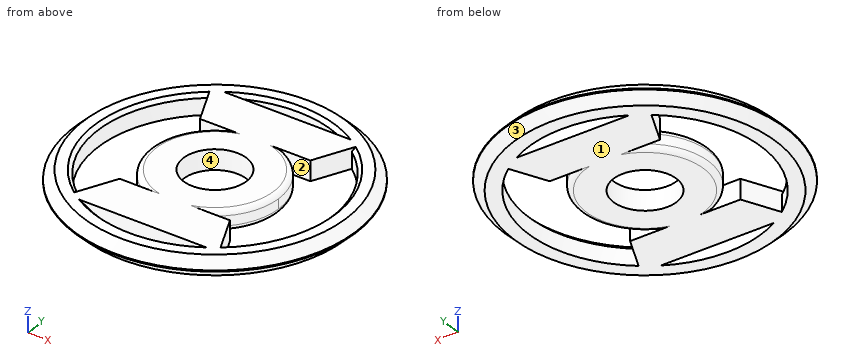
```python
from build123d import *

# Parameters (mm, degrees)
F0_R         = 49.0432335283
F0_R_2       = 10.9855
F1_DEPTH     = 6.985
F2_T4_ANGLE  = 164.4789683114
F2_T10_ANGLE = 164.4789683114
F2_T16_ANGLE = 164.4789683114
F2_T22_ANGLE = 164.4789683114
F3_T4_ANGLE  = 113.2359316918
F3_T10_ANGLE = 67.3888483325
F3_T15_ANGLE = 113.2359316918
F3_T21_ANGLE = 67.3888483325
F4_SIZE      = 3.302


# Not quite as in the source:
# - a fillet or chamfer that OpenCascade refuses, or shapes differently, is made with other operations: its cross-section is extruded or revolved along the edge and cut away or added


with BuildPart() as f1:
    # F0 (on Top) → F1 (new body)
    with BuildSketch(Plane.XY):
        Circle(F0_R)
        with BuildLine():
            Line((26.67, 35.56), (25.0451862182, 32.0755756003))
            ThreePointArc((25.0451862182, 32.0755756003), (36.5740630803, 17.8449380104), (40.6952565147, 0))
            ThreePointArc((40.6952565147, 0), (36.5738989199, -17.8452744611), (25.0445960757, -32.0760363854))
            Line((25.0445960757, -32.0760363854), (26.67, -35.56))
            Line((26.67, -35.56), (19.7886407516, -35.56))
            ThreePointArc((19.7886407516, -35.56), (0, -40.6952565147), (-19.7886407516, -35.56))
            Line((-19.7886407516, -35.56), (-26.67, -35.56))
            Line((-26.67, -35.56), (-25.0445960757, -32.0760363854))
            ThreePointArc((-25.0445960757, -32.0760363854), (-40.695256513, -0.0003743631), (-25.0451862182, 32.0755756003))
            Line((-25.0451862182, 32.0755756003), (-26.67, 35.56))
            Line((-26.67, 35.56), (-19.7886407516, 35.56))
            ThreePointArc((-19.7886407516, 35.56), (0, 40.6952565147), (19.7886407516, 35.56))
            Line((19.7886407516, 35.56), (26.67, 35.56))
        make_face(mode=Mode.SUBTRACT)
        with BuildLine():
            ThreePointArc((-10.1860168797, 19.7533714876), (0, 22.225), (10.1860168797, 19.7533714876))
            Line((10.1860168797, 19.7533714876), (19.299248075, 19.7533714876))
            Line((19.299248075, 19.7533714876), (25.0451862182, 32.0755756003))
            ThreePointArc((25.0451862182, 32.0755756003), (22.4845127485, 33.9197669399), (19.7886407516, 35.56))
            Line((19.7886407516, 35.56), (-19.7886407516, 35.56))
            ThreePointArc((-19.7886407516, 35.56), (-22.4845127485, 33.9197669399), (-25.0451862182, 32.0755756003))
            Line((-25.0451862182, 32.0755756003), (-19.299248075, 19.7533714876))
            Line((-19.299248075, 19.7533714876), (-10.1860168797, 19.7533714876))
        make_face()
        with BuildLine():
            Line((-26.67, 35.56), (-25.0451862182, 32.0755756003))
            ThreePointArc((-25.0451862182, 32.0755756003), (-22.4845127485, 33.9197669399), (-19.7886407516, 35.56))
            Line((-19.7886407516, 35.56), (-26.67, 35.56))
        make_face()
        with BuildLine():
            ThreePointArc((19.7886407516, 35.56), (22.4845127485, 33.9197669399), (25.0451862182, 32.0755756003))
            Line((25.0451862182, 32.0755756003), (26.67, 35.56))
            Line((26.67, 35.56), (19.7886407516, 35.56))
        make_face()
        with BuildLine():
            ThreePointArc((10.1708209875, -19.7612), (18.9736280327, -11.5737662097), (22.225, 0))
            ThreePointArc((22.225, 0), (18.9780774863, 11.5664687751), (10.1860168797, 19.7533714876))
            Line((10.1860168797, 19.7533714876), (0, 19.7533714876))
            Line((0, 19.7533714876), (-10.1860168797, 19.7533714876))
            ThreePointArc((-10.1860168797, 19.7533714876), (-22.2249983566, -0.0085469402), (-10.1708209875, -19.7612))
            Line((-10.1708209875, -19.7612), (0, -19.7612))
            Line((0, -19.7612), (10.1708209875, -19.7612))
        make_face()
        Circle(F0_R_2, mode=Mode.SUBTRACT)
        with BuildLine():
            Line((0, 19.7533714876), (10.1860168797, 19.7533714876))
            ThreePointArc((10.1860168797, 19.7533714876), (0, 22.225), (-10.1860168797, 19.7533714876))
            Line((-10.1860168797, 19.7533714876), (0, 19.7533714876))
        make_face()
        with BuildLine():
            Line((19.299248075, -19.7612), (10.1708209875, -19.7612))
            ThreePointArc((10.1708209875, -19.7612), (0, -22.225), (-10.1708209875, -19.7612))
            Line((-10.1708209875, -19.7612), (-19.299248075, -19.7612))
            Line((-19.299248075, -19.7612), (-25.0445960757, -32.0760363854))
            ThreePointArc((-25.0445960757, -32.0760363854), (-22.4842007134, -33.9199737776), (-19.7886407516, -35.56))
            Line((-19.7886407516, -35.56), (19.7886407516, -35.56))
            ThreePointArc((19.7886407516, -35.56), (22.4842007134, -33.9199737776), (25.0445960757, -32.0760363854))
            Line((25.0445960757, -32.0760363854), (19.299248075, -19.7612))
        make_face()
        with BuildLine():
            ThreePointArc((-10.1708209875, -19.7612), (0, -22.225), (10.1708209875, -19.7612))
            Line((10.1708209875, -19.7612), (0, -19.7612))
            Line((0, -19.7612), (-10.1708209875, -19.7612))
        make_face()
        with BuildLine():
            ThreePointArc((-19.7886407516, -35.56), (-22.4842007134, -33.9199737776), (-25.0445960757, -32.0760363854))
            Line((-25.0445960757, -32.0760363854), (-26.67, -35.56))
            Line((-26.67, -35.56), (-19.7886407516, -35.56))
        make_face()
        with BuildLine():
            Line((26.67, -35.56), (25.0445960757, -32.0760363854))
            ThreePointArc((25.0445960757, -32.0760363854), (22.4842007134, -33.9199737776), (19.7886407516, -35.56))
            Line((19.7886407516, -35.56), (26.67, -35.56))
        make_face()
    extrude(amount=F1_DEPTH)

    # F2: fillet of radius 1.778 on 4 edges, made by hand


with BuildPart() as f2_tool2:
    # F2_s3 → F2_t4 (revolve)
    with BuildSketch(Plane(origin=(0, 0, 0), x_dir=(0, 0, 1), z_dir=(0.9907891286, 0.1354138197, 0))):
        with BuildLine():
            ThreePointArc((5.207, -22.225), (6.4642358569, -21.7042358569), (6.985, -20.447))
            Line((6.985, -20.447), (6.985, -22.225))
            Line((6.985, -22.225), (5.207, -22.225))
        make_face()
    revolve(axis=Axis((0, 0, 6.985), (0, 0, 1)), revolution_arc=F2_T4_ANGLE)

    split(bisect_by=Plane.XZ.offset(-19.7533714876), keep=Keep.TOP)

    split(bisect_by=Plane.XZ.offset(19.7612), keep=Keep.BOTTOM)


with BuildPart() as f1_1:
    add(f1.part)

    # F2_t1: cut F2_tool2
    add(f2_tool2.part, mode=Mode.SUBTRACT)


with BuildPart() as f2_tool8:
    # F2_s9 → F2_t10 (revolve)
    with BuildSketch(Plane(origin=(0, 0, 0), x_dir=(0, 0, 1), z_dir=(-0.9908929862, -0.1346517356, 0))):
        with BuildLine():
            ThreePointArc((5.207, -22.225), (6.4642358569, -21.7042358569), (6.985, -20.447))
            Line((6.985, -20.447), (6.985, -22.225))
            Line((6.985, -22.225), (5.207, -22.225))
        make_face()
    revolve(axis=Axis((0, 0, 6.985), (0, 0, 1)), revolution_arc=F2_T10_ANGLE)

    split(bisect_by=Plane.XZ.offset(19.7612), keep=Keep.BOTTOM)

    split(bisect_by=Plane.XZ.offset(-19.7533714876), keep=Keep.TOP)


with BuildPart() as f1_2:
    add(f1_1.part)

    # F2_t7: cut F2_tool8
    add(f2_tool8.part, mode=Mode.SUBTRACT)


with BuildPart() as f2_tool14:
    # F2_s15 → F2_t16 (revolve)
    with BuildSketch(Plane(origin=(0, 0, 0), x_dir=(0, 0, 1), z_dir=(-0.9908929862, -0.1346517356, 0))):
        with BuildLine():
            ThreePointArc((1.778, -22.225), (0.5207641431, -21.7042358569), (0, -20.447))
            Line((0, -20.447), (0, -22.225))
            Line((0, -22.225), (1.778, -22.225))
        make_face()
    revolve(axis=Axis((0, 0, 0), (0, 0, 1)), revolution_arc=F2_T16_ANGLE)

    split(bisect_by=Plane.XZ.offset(19.7612), keep=Keep.BOTTOM)

    split(bisect_by=Plane.XZ.offset(-19.7533714876), keep=Keep.TOP)


with BuildPart() as f1_3:
    add(f1_2.part)

    # F2_t13: cut F2_tool14
    add(f2_tool14.part, mode=Mode.SUBTRACT)


with BuildPart() as f2_tool20:
    # F2_s21 → F2_t22 (revolve)
    with BuildSketch(Plane(origin=(0, 0, 0), x_dir=(0, 0, 1), z_dir=(0.9907891286, 0.1354138197, 0))):
        with BuildLine():
            ThreePointArc((1.778, -22.225), (0.5207641431, -21.7042358569), (0, -20.447))
            Line((0, -20.447), (0, -22.225))
            Line((0, -22.225), (1.778, -22.225))
        make_face()
    revolve(axis=Axis((0, 0, 0), (0, 0, 1)), revolution_arc=F2_T22_ANGLE)

    split(bisect_by=Plane.XZ.offset(-19.7533714876), keep=Keep.TOP)

    split(bisect_by=Plane.XZ.offset(19.7612), keep=Keep.BOTTOM)


with BuildPart() as f1_4:
    add(f1_3.part)

    # F2_t19: cut F2_tool20
    add(f2_tool20.part, mode=Mode.SUBTRACT)

    # F3: chamfer of 1.27 on 4 edges, made by hand


with BuildPart() as f3_tool2:
    # F3_s3 → F3_t4 (revolve)
    with BuildSketch(Plane(origin=(0, 0, 0), x_dir=(0, 0, 1), z_dir=(0.8350254942, -0.550211254, 0))):
        Polygon((6.985, 41.9652565147), (5.715, 40.6952565147), (6.985, 40.6952565147), align=None)
    revolve(axis=Axis((0, 0, 6.985), (0, 0, -1)), revolution_arc=F3_T4_ANGLE)

    split(bisect_by=Plane(origin=(-8.2863025765, -3.8639663492, 0), x_dir=(0, 0, 1), z_dir=(-0.906307787, -0.4226182617, 0)), keep=Keep.TOP)

    split(bisect_by=Plane(origin=(-8.2780879413, 3.8620485498, 0), x_dir=(0, 0, 1), z_dir=(-0.906227568, 0.4227902494, 0)), keep=Keep.TOP)


with BuildPart() as f1_5:
    add(f1_4.part)

    # F3_t1: cut F3_tool2
    add(f3_tool2.part, mode=Mode.SUBTRACT)


with BuildPart() as f3_tool8:
    # F3_s9 → F3_t10 (revolve)
    with BuildSketch(Plane(origin=(0, 0, 0), x_dir=(0, 0, 1), z_dir=(-0.8320081138, -0.5547634618, 0))):
        Polygon((6.985, 41.9652565147), (5.715, 40.6952565147), (6.985, 40.6952565147), align=None)
    revolve(axis=Axis((0, 0, 6.985), (0, 0, -1)), revolution_arc=F3_T10_ANGLE)

    split(bisect_by=Plane.XZ.offset(-35.56), keep=Keep.BOTTOM)


with BuildPart() as f1_6:
    add(f1_5.part)

    # F3_t7: cut F3_tool8
    add(f3_tool8.part, mode=Mode.SUBTRACT)


with BuildPart() as f3_tool13:
    # F3_s14 → F3_t15 (revolve)
    with BuildSketch(Plane(origin=(0, 0, 0), x_dir=(0, 0, 1), z_dir=(-0.8350153711, 0.550226617, 0))):
        Polygon((6.985, 41.9652565147), (5.715, 40.6952565147), (6.985, 40.6952565147), align=None)
    revolve(axis=Axis((0, 0, 6.985), (0, 0, -1)), revolution_arc=F3_T15_ANGLE)

    split(bisect_by=Plane(origin=(8.2780879413, 3.8620485498, 0), x_dir=(0, 0, 1), z_dir=(0.906227568, 0.4227902494, 0)), keep=Keep.TOP)

    split(bisect_by=Plane(origin=(8.2863025765, -3.8639663492, 0), x_dir=(0, 0, 1), z_dir=(0.906307787, -0.4226182617, 0)), keep=Keep.TOP)


with BuildPart() as f1_7:
    add(f1_6.part)

    # F3_t12: cut F3_tool13
    add(f3_tool13.part, mode=Mode.SUBTRACT)


with BuildPart() as f3_tool19:
    # F3_s20 → F3_t21 (revolve)
    with BuildSketch(Plane(origin=(0, 0, 0), x_dir=(0, 0, 1), z_dir=(0.8320081138, 0.5547634618, 0))):
        Polygon((6.985, 41.9652565147), (5.715, 40.6952565147), (6.985, 40.6952565147), align=None)
    revolve(axis=Axis((0, 0, 6.985), (0, 0, -1)), revolution_arc=F3_T21_ANGLE)

    split(bisect_by=Plane.XZ.offset(35.56), keep=Keep.TOP)


with BuildPart() as f1_8:
    add(f1_7.part)

    # F3_t18: cut F3_tool19
    add(f3_tool19.part, mode=Mode.SUBTRACT)

    # F4
    f4_edges = [f1_8.edges().sort_by_distance(p)[0] for p in [
        (-49.043234, 0, 6.985),
        (-49.043234, 0, 0),
    ]]
    chamfer(f4_edges, length=F4_SIZE)


solid = f1_8.part
```
Source: CAD feature listing. Evaluate the final solid. Frame: model axes, mm. Face numbers are marked on the shaded views. Coordinates: 2 decimals unless noted, no trailing zeros. Answer as CSV lines item,"result".
1. Mould query, pull axis Y, two halves, no side actions, for the marked faces 1, 2, 3 and 4. Classes: released by +Y, released by -Y, zero draft, split by the parting line, or undercut.
Established:
face 1,"zero draft"
face 2,"undercut"
face 3,"split by the parting line"
face 4,"undercut"
2. Ray query, line 1 (Y direction, x = 0, z = 3.5); line 2 (X direction, y = 22.5, z = 2.5); line 3 (X direction, y = -4.5, z = 1.75). Return the intervals inside material, ascending.
Established:
line 1,"y = -49.04 to -40.7, -35.56 to -10.99, 10.99 to 35.56, 40.7 to 49.04"
line 2,"x = -42.67 to -33.91, -20.58 to 20.58, 33.91 to 42.67"
line 3,"x = -47.28 to -40.45, -21.76 to -10.02, 10.02 to 21.76, 40.45 to 47.28"
3. Section A-A (x = 0). Count the separate pieces of the cut face and the enclosed holes in it, then the cut area to 3 significant figures.
Established:
separate pieces,"4"
enclosed holes,"0"
area,"437 mm2"
4. Contact query for flat-ended pins moving along their axis: pin 1 (1 mm diameter, centred on x = -32, y = -24, fed in from +Z); pin 2 (3.5 mm diameter, centred on x = 9.5, z = 3.5, fed in from +Y); pin 3 (1.5 mm diameter, centred on x = -0.5, z = 2, fed in from -Y); pin 4 (2 mm diameter, centred on x = 35, z = 3.5, fed in from +Y). Output: stop coordinate, or through.
Established:
pin 1,"passes through"
pin 2,"stops at y = 48.43"
pin 3,"stops at y = -48.49"
pin 4,"stops at y = 35.34"
